from build123d import *

# Parameters (mm, degrees)
SKETCH1_W           = 13
SKETCH1_H           = 13
BOSS_EXTRUDE1_DEPTH = 40
CUT_EXTRUDE1_DEPTH  = 43.558782877
SKETCH3_R           = 2
SKETCH3_R_2         = 2.5
CUT_EXTRUDE2_DEPTH  = 43.558782877
SKETCH5_W           = 13
SKETCH5_H           = 13
BOSS_EXTRUDE2_DEPTH = 1
FILLET1_R           = 1


with BuildPart() as part:
    # Sketch1 → Boss-Extrude1 (new, symmetric)
    with BuildSketch(Plane.XY):
        Rectangle(SKETCH1_W, SKETCH1_H)
    extrude(amount=BOSS_EXTRUDE1_DEPTH, both=True)

    # Sketch2 → Cut-Extrude1 (cut, through all)
    with BuildSketch(Plane(origin=(0, 6.5, 0), x_dir=(1, 0, 0), z_dir=(0, 1, 0))):
        with BuildLine():
            ThreePointArc((3.570714214, 0), (0, 8.5), (-3.570714214, 0))
            ThreePointArc((-3.570714214, 0), (0, -8.5), (3.570714214, 0))
        make_face()
    extrude(amount=-CUT_EXTRUDE1_DEPTH, mode=Mode.SUBTRACT)

    # Sketch3 → Cut-Extrude2 (cut, through all)
    with BuildSketch(Plane(origin=(6.5, 0, 0), x_dir=(0, 0, -1), z_dir=(1, 0, 0))):
        with Locations((-35, 0)):
            Circle(SKETCH3_R)
        with Locations((-24, 0)):
            Circle(SKETCH3_R)
        with Locations((20, 0)):
            Circle(SKETCH3_R_2)
        with Locations((35, 0)):
            Circle(SKETCH3_R_2)
    extrude(amount=-CUT_EXTRUDE2_DEPTH, mode=Mode.SUBTRACT)

    # Sketch5 → Boss-Extrude2 (add)
    with BuildSketch(Plane.ZY.offset(6.5)):
        Rectangle(SKETCH5_W, SKETCH5_H)
    extrude(amount=BOSS_EXTRUDE2_DEPTH)

    # Fillet1
    fillet1_edges = [part.edges().sort_by_distance(p)[0] for p in [
        (-7, -6.5, 6.5),
        (-7, 6.5, 6.5),
        (-7, 6.5, -6.5),
        (-7, -6.5, -6.5),
    ]]
    fillet(fillet1_edges, radius=FILLET1_R)


solid = part.part
Check sheet for the modelled part. Datum: model origin and axes. Units: mm. Coordinates: 2 decimals unless noted, no trailing zeros. Loops run counter-clockwise (first coordinate to the right, second up) from the corner with the lowest first, then second, coordinate; pieces in that order, holes last. Notation, with made-up numbers: (69, 36) -> (120, 36) arc R15 ccw to (120, 57) -> close; hole circle Ø1 at (86.5, 76). An arc over 180 degrees is marked (long way). Answer in a Markdown table with one row per item.
1. Sectioned sample at D-D, the plane y = -4. Record the boundary of the cut face in (x, z), then the cut area to 3 significant figures.
Check values:
| item | result |
|---|---|
| outline | (-7.5, -6.5) -> (-6.5, -6.5) -> (-6.5, -40) -> (6.5, -40) -> (6.5, 40) -> (-6.5, 40) -> (-6.5, 6.5) -> (-7.5, 6.5) -> close; hole (-3.57, 0) arc R5 ccw (long way) to (3.57, 0) arc R5 ccw (long way) to start |
| area | 911 mm2 |
2. Material ranges on line 1 along Y through (x, z) = (3, 24); line 2 along Z through (x, y) = (0, -1.75); line 3 along Y through (x, z) = (-0.75, -35), recorded low to high. Write a range as [from, to].
Check values:
| item | result |
|---|---|
| line 1 | y = [-6.5, -2], [2, 6.5] |
| line 2 | z = [-40, -36.79], [-33.21, -21.79], [-18.21, -8.5], [8.5, 23.03], [24.97, 34.03], [35.97, 40] |
| line 3 | y = [-6.5, -2.5], [2.5, 6.5] |
3. Sectioned sample at C-C, the plane y = 0. Record the boundary of the cut face in (x, z), then the cut area to 3 significant figures.
Check values:
| item | result |
|---|---|
| outline | (-7.5, -6.5) -> (-6.5, -6.5) -> (-6.5, -17.5) -> (6.5, -17.5) -> (6.5, 22) -> (-6.5, 22) -> (-6.5, 6.5) -> (-7.5, 6.5) -> close; (-6.5, -40) -> (6.5, -40) -> (6.5, -37.5) -> (-6.5, -37.5) -> close; (-6.5, -32.5) -> (6.5, -32.5) -> (6.5, -22.5) -> (-6.5, -22.5) -> close; (-6.5, 26) -> (6.5, 26) -> (6.5, 33) -> (-6.5, 33) -> close; (-6.5, 37) -> (6.5, 37) -> (6.5, 40) -> (-6.5, 40) -> close; hole (-3.57, 0) arc R5 ccw (long way) to (3.57, 0) arc R5 ccw (long way) to start |
| area | 677 mm2 |
4. Sectioned sample at A-A, the plane x = 0. Record the boundary of the cut face in (y, z), then the cut area to 3 significant figures.
Check values:
| item | result |
|---|---|
| outline | (-6.5, -40) -> (6.5, -40) -> (6.5, -8.5) -> (-6.5, -8.5) -> close; (-6.5, 8.5) -> (6.5, 8.5) -> (6.5, 40) -> (-6.5, 40) -> close; hole circle Ø5 at (0, -35); hole circle Ø5 at (0, -20); hole circle Ø4 at (0, 24); hole circle Ø4 at (0, 35) |
| area | 755 mm2 |
5. Go/stop test with flat-tipped pins: pin 1 (8 mm diameter, centred on x = 0, z = 3.5, fed in from -Y); pin 2 (0.5 mm diameter, centred on x = -7, y = 1, fed in from -Z). Record where each tip stops, or that it passes through.
Check values:
| item | result |
|---|---|
| pin 1 | passes through |
| pin 2 | stops at z = -6.5 |
6. Sectioned sample at B-B, the plane z = -35. Record the boundary of the cut face in (x, y).
Check values:
| item | result |
|---|---|
| outline | (-6.5, -6.5) -> (6.5, -6.5) -> (6.5, -2.5) -> (-6.5, -2.5) -> close; (-6.5, 2.5) -> (6.5, 2.5) -> (6.5, 6.5) -> (-6.5, 6.5) -> close |
7. Release check for a two-part mould opening along Y. For faces 1 (the face through (0.09, -0.96, -37.31)), 2 (the face through (-5, -6.5, 1)), 3 (the face through (0, 0, 26)), 4 (the face through (0, 0, -40)) record: released by +Y, released by -Y, zero draft, split by the parting line, or undercut.
Check values:
| item | result |
|---|---|
| face 1 | undercut |
| face 2 | released by -Y |
| face 3 | undercut |
| face 4 | zero draft |
